from build123d import *

# Parameters (mm, degrees)
SKETCH1_R           = 11
BOSS_EXTRUDE1_DEPTH = 3.5
SKETCH2_R           = 4.1
CUT_EXTRUDE3_DEPTH  = 3
CIRPATTERN1_COUNT   = 8


with BuildPart() as part:
    # Sketch1 → Boss-Extrude1 (new body, symmetric)
    with BuildSketch(Plane.XY):
        Polygon((6.213203436, 15), (-6.213203436, 15), (-15, 6.213203436), (-15, -6.213203436), (-6.213203436, -15), (6.213203436, -15), (15, -6.213203436), (15, 6.213203436), align=None)
        Circle(SKETCH1_R, mode=Mode.SUBTRACT)
    extrude(amount=BOSS_EXTRUDE1_DEPTH, both=True)

    # Sketch2 → Cut-Extrude3 (cut)
    with BuildSketch(Plane(origin=(0, -15, 0), x_dir=(-1, 0, 0), z_dir=(0, -1, 0))):
        Circle(SKETCH2_R)
    cut_extrude3 = extrude(amount=-CUT_EXTRUDE3_DEPTH, mode=Mode.SUBTRACT)

    # CirPattern1: Cut-Extrude3 ×8 about axis
    cirpattern1_axis = Axis((0, 0, 0), (0, 0, 1))
    for i in range(1, CIRPATTERN1_COUNT):
        add(cut_extrude3.rotate(cirpattern1_axis, i * 360 / CIRPATTERN1_COUNT), mode=Mode.SUBTRACT)


solid = part.part
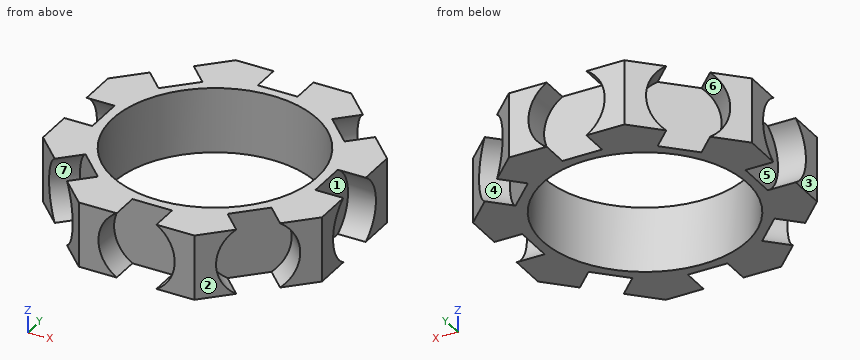
Could you check a few things on this model? Use its own coordinates, in mm. Face numbers are marked on the shaded views. A direction names the side the tool comes from. Give positions to 0.01 mm unless a question says otherwise; leave off trailing zeros. Write each loop counter-clockwise with the first axis right and the second up, starting at its lowest first coordinate (ties: lowest second). Pieces come first, ordered by that corner, then holes. Notation, with made-up numbers: (40, 49) -> (80, 49) arc R13 ccw to (80, 59) -> close; hole circle Ø5 at (44.25, -37). An arc over 180 degrees is marked (long way). Answer as CSV lines item,"result". Start each with the question number.
(1) If we mould it in two halves opening along Y, with no side actions, what happens to the marked faces 1, 2, 3 and 4? For each: +Y half, -Y half, draft (parallel to the pull), parting line (faces both ways), or undercut.
(2) If we section it at A-A, the plane x = 0: Write out the boundary of the cut face in (y, z), and give its area (3 significant figures).
(3) If we section it at C-C, the plane y = 8.5: Give the number of separate pieces and of enclosed holes in the cut face, and give its area (3 significant figures).
(4) Which directions (+Z, -Z, +X, -X, +Y, -Y) give clear straight access to the entire face, cutting with the end or side of a thin tool? Please do the marked faces 5, 6 and 7.
(5) I'm going to push flat-ended pins straight in: pin 1 Ø2 at (x, z) = (0.5, 0) entering from -Y; pin 2 Ø3.5 at (y, z) = (-0.5, 0.5) entering from +X. Where does each tip first touch, or does it pass through?
(6) Please list where these lines run through material, in increasing order: line 1 (Y direction, x = 0, z = 0.5); line 2 (Z direction, x = -13, y = -3.5); line 3 (X direction, y = -9.5, z = 2).
Answer list:
1,face 1,"undercut"
1,face 2,"-Y half"
1,face 3,"draft"
1,face 4,"+Y half"
2,outline,"(-12, -3.5) -> (-11, -3.5) -> (-11, 3.5) -> (-12, 3.5) -> close; (11, -3.5) -> (12, -3.5) -> (12, 3.5) -> (11, 3.5) -> close"
2,area,"14.0 mm^2"
3,separate pieces,"6"
3,enclosed holes,"0"
3,area,"22.3 mm^2"
4,face 5,"-X"
4,face 6,"+Y"
4,face 7,"-Y"
5,pin 1,"y = -12"
5,pin 2,"x = 12"
6,line 1,"-12 to -11, 11 to 12"
6,line 2,"-3.5 to -2.14, 2.14 to 3.5"
6,line 3,"-7.47 to -5.55, 5.55 to 7.47"
